from build123d import *

# Parameters (mm, degrees)
F0_W      = 131.6228
F0_H      = 90.3224
F1_DEPTH  = 3
F2_W      = 123.6228
F2_H      = 82.3224
F3_DEPTH  = 3
F3_TAPER  = 5
F4_W      = 17
F4_H      = 3
F5_DEPTH  = 5
F6_W      = 3
F6_H      = 5
F7_DEPTH  = 4
F8_R      = 3
F10_DEPTH = 25


with BuildPart() as f1:
    # F0 (on Top) → F1 (new body)
    with BuildSketch(Plane.XY):
        Rectangle(F0_W, F0_H)
    extrude(amount=F1_DEPTH)

    # F2 (on face) → F3 (join)
    with BuildSketch(Plane(origin=(0, 0, 0), x_dir=(1, 0, 0), z_dir=(0, 0, -1))):
        Rectangle(F2_W, F2_H)
    extrude(amount=F3_DEPTH, taper=F3_TAPER)

    # F4 (on face) → F5 (join)
    with BuildSketch(Plane(origin=(0, 45.1612, 0), x_dir=(-1, 0, 0), z_dir=(0, 1, 0))):
        with Locations((35, 1.5)):
            Rectangle(F4_W, F4_H)
        with Locations((-35, 1.5)):
            Rectangle(F4_W, F4_H)
    extrude(amount=F5_DEPTH)

    # F6 (on face) → F7 (join)
    with BuildSketch(Plane(origin=(0, 0, 0), x_dir=(1, 0, 0), z_dir=(0, 0, -1))):
        with Locations((-42, -47.6612)):
            Rectangle(F6_W, F6_H)
        with Locations((-28, -47.6612)):
            Rectangle(F6_W, F6_H)
        with Locations((28, -47.6612)):
            Rectangle(F6_W, F6_H)
        with Locations((42, -47.6612)):
            Rectangle(F6_W, F6_H)
    extrude(amount=F7_DEPTH)

    # F8
    f8_edges = [f1.edges().sort_by_distance(p)[0] for p in [
        (-42, 45.1612, -4),
        (-28, 45.1612, -4),
    ]]
    fillet(f8_edges, radius=F8_R)

    # F9 (on face) → F10 (cut)
    with BuildSketch(Plane(origin=(-43.5, 0, 0), x_dir=(0, -1, 0), z_dir=(-1, 0, 0))):
        with BuildLine():
            Line((-45.1612, -1), (-45.1612, 0))
            Line((-45.1612, 0), (-45.6612, 0))
            Line((-45.6612, 0), (-45.6612, -2.6583123952))
            ThreePointArc((-45.6612, -2.6583123952), (-45.2889186767, -1.8660254038), (-45.1612, -1))
        make_face()
    extrude(amount=-F10_DEPTH, mode=Mode.SUBTRACT)

    # F11 (on face) → F12 (revolve)
    with BuildSketch(Plane.YZ.offset(-40.5)):
        with BuildLine():
            Line((47.0152064206, -1.9), (49.5071935794, -1.9))
            ThreePointArc((49.5071935794, -1.9), (48.2612, -0.75), (47.0152064206, -1.9))
        make_face()
    revolve(axis=Axis((-40.5, 47.9112, -2), (0, -1, 0)))

    # F13 (on face) → F14 (revolve)
    with BuildSketch(Plane(origin=(-29.5, 0, 0), x_dir=(0, -1, 0), z_dir=(-1, 0, 0))):
        with BuildLine():
            Line((-49.5112, -1.9), (-47.0192128411, -1.9))
            ThreePointArc((-47.0192128411, -1.9), (-48.2652064206, -0.75), (-49.5112, -1.9))
        make_face()
    revolve(axis=Axis((-29.5, 47.9112, -2), (0, 1, 0)))


solid = f1.part
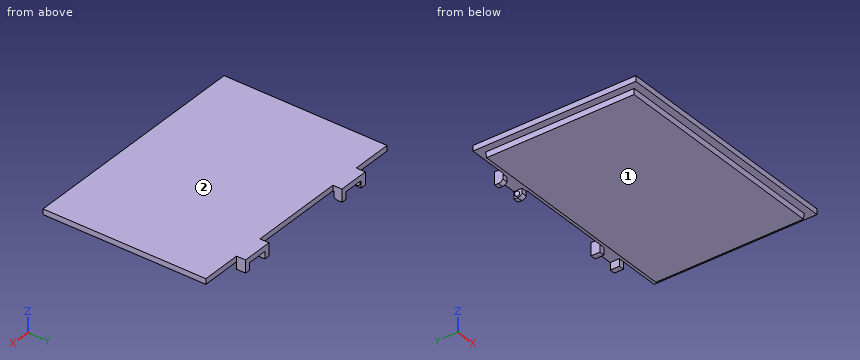
Could you check a few things on this model? Use its own coordinates, in mm. Face numbers are marked on the shaded views. A direction names the side the tool comes from. Give positions to 0.01 mm unless a question says otherwise; leave off trailing zeros.
1. For the marked faces 1 and 2, which set-ups out of +Z, -Z, +X, -X, +Y, -Y let a thin tool reach every point of the face, with its end or its side?
2. Will these pins go through, and if not, where does the flat tip stop? P1, Ø1.5, axis at x = 58, z = 2, coming from the +Y side; P2, Ø8, axis at x = 0.5, y = -27.5, coming from the -Z side; P3, Ø3, axis at y = 48, z = -2.5, coming from the +X side.
3. I need wall thicknesses on L1, parallel to Y at x = 52, z = 2.25; L2, parallel to Y at x = -43, z = -2.25; L3, parallel to Z at x = 34.5, y = -39. Which ranges of each line are inside material? Lowest first, please.
Solved:
1. face 1: -Z, +X, -X, -Y
1. face 2: +Z, +X, -X, +Y, -Y
2. P1: stops at y = 45.16
2. P2: stops at z = -3
2. P3: stops at x = 43.5
3. L1: y = -45.16 to 45.16
3. L2: y = -40.96 to 40.96, 45.66 to 50.16
3. L3: z = -3 to 3
